Input: part model. Units: mm. Frame: model coordinates. A direction names the side the tool comes from. Round coordinates to 2 decimals unless told otherwise and drop trailing zeros. Loops run counter-clockwise (first coordinate to the right, second up) from the corner with the lowest first, then second, coordinate; pieces in that order, holes last. Notation, with made-up numbers: M 53.25,52 L 63.25,52 A8 ccw 63.25,60 Z; hole C -38.5,17 d6. An arc over 180 degrees is marked long. Use one line per item in the form item = value. Start each with the question number.
Q1. Ray query, line 1 along X through (y, z) = (0.75, -5.75); line 2 along Y through (x, z) = (4.25, 2); line 3 along Y through (x, z) = (-1, -2.5). Return the intervals inside material, ascending.
Q2. Section query D-D, the plane z = -0.85. Output: boundary loops of the cut face in (x, y), and give its area (3 significant figures).
Q3. Section query C-C, the plane y = 6.75. Output: boundary loops of the cut face in (x, z), and give its area (3 significant figures).
Q4. Mould query, pull axis X, two halves, no side actions, for faces 3 (the cylindrical face through (-7.134, 0.811, 5.536)), 4 (the flat face through (-2.5, 3, -1)), 5 (the flat face through (2, -0.01, 6)). Classes: pulls with the +X half, pulls with the -X half, needs draft (parallel to the pull), parting line crosses it, or undercut.
Q5. Access query for faces 1 (the flat face through (-7, -0.01, 6)), 2 (the flat face through (0, 3.6, -1)). Directions: +Z, -Z, +X, -X, +Y, -Y. A direction counts if a zero-diameter tool reaches every point of the face in a straight line with its end or side. Return the directions, or none.
Q6. Section query B-B, the plane z = -5.75. State how many separate pieces and enclosed holes the cut face has, and give its area (3 significant figures).
Q7. First-contact query: P1, Ø8.5, axis at x = 4.5, z = 2.5, coming from the +Y side; P2, Ø1.2, axis at x = 6.5, z = -6, coming from the +Y side; P3, Ø1.4, axis at x = -5, z = 6, coming from the +Y side; P4, Ø3, axis at x = 0, z = -5.5, coming from the -Y side. Flat tips, straight axial feed; report the tip coordinate or a pass-through.
```python
from build123d import *

# Parameters (mm, degrees)
BOSS_EXTRUDE1_DEPTH = 1.6
SKETCH2_R           = 1.1
SKETCH2_R_2         = 0.5
CUT_EXTRUDE1_DEPTH  = 1.6
SKETCH3_R           = 1.2
SKETCH3_R_2         = 1.09
SKETCH3_R_3         = 0.9
SKETCH3_R_4         = 0.49
BOSS_EXTRUDE2_DEPTH = 1.62
SKETCH5_W           = 5
SKETCH5_H           = 5
BOSS_EXTRUDE3_DEPTH = 2
SKETCH6_R           = 1.25
SKETCH6_R_2         = 0.95
BOSS_EXTRUDE4_DEPTH = 3.6


with BuildPart() as part:
    # Sketch1 → Boss-Extrude1 (new body)
    with BuildSketch(Plane(origin=(0, 0, 0), x_dir=(1, 0, 0), z_dir=(0, 1, 0))):
        with BuildLine():
            Line((-6.89, 8.35), (6.89, 8.35))
            ThreePointArc((6.89, 8.35), (8.304213562, 7.764213562), (8.89, 6.35))
            Line((8.89, 6.35), (8.89, -6.35))
            ThreePointArc((8.89, -6.35), (8.304213562, -7.764213562), (6.89, -8.35))
            Line((6.89, -8.35), (-6.89, -8.35))
            ThreePointArc((-6.89, -8.35), (-8.304213562, -7.764213562), (-8.89, -6.35))
            Line((-8.89, -6.35), (-8.89, 6.35))
            ThreePointArc((-8.89, 6.35), (-8.304213562, 7.764213562), (-6.89, 8.35))
        make_face()
    extrude(amount=BOSS_EXTRUDE1_DEPTH)

    # Sketch2 → Cut-Extrude1 (cut)
    with BuildSketch(Plane(origin=(0, 1.6, 0), x_dir=(1, 0, 0), z_dir=(0, 1, 0))):
        with Locations(Location((-6.29, 5.75, 0), (0, 0, 270))):
            Circle(SKETCH2_R)
        with Locations(Location((6.29, 5.75, 0), (0, 0, 90))):
            Circle(SKETCH2_R)
        with Locations(Location((-7.62, -5.6, 0), (0, 0, 270))):
            Circle(SKETCH2_R_2)
        with Locations(Location((-5.08, -5.6, 0), (0, 0, 270))):
            Circle(SKETCH2_R_2)
        with Locations(Location((-2.54, -5.6, 0), (0, 0, 270))):
            Circle(SKETCH2_R_2)
        with Locations(Location((0, -5.6, 0), (0, 0, 270))):
            Circle(SKETCH2_R_2)
        with Locations(Location((2.54, -5.6, 0), (0, 0, 270))):
            Circle(SKETCH2_R_2)
        with Locations(Location((5.08, -5.6, 0), (0, 0, 270))):
            Circle(SKETCH2_R_2)
        with Locations(Location((7.62, -5.6, 0), (0, 0, 270))):
            Circle(SKETCH2_R_2)
    extrude(amount=-CUT_EXTRUDE1_DEPTH, mode=Mode.SUBTRACT)

    # Sketch3 → Boss-Extrude2 (add)
    # profile 1 of 9: a face of its own
    with BuildSketch(Plane(origin=(0, 1.61, 0), x_dir=(1, 0, 0), z_dir=(0, 1, 0))):
        with Locations(Location((-6.29, 5.75, 0), (0, 0, 270))):
            Circle(SKETCH3_R)
        with Locations(Location((-6.29, 5.75, 0), (0, 0, 270))):
            Circle(SKETCH3_R_2, mode=Mode.SUBTRACT)
    # profile 2 of 9: a face of its own
    with BuildSketch(Plane(origin=(0, 1.61, 0), x_dir=(1, 0, 0), z_dir=(0, 1, 0))):
        with Locations(Location((6.29, 5.75, 0), (0, 0, 270))):
            Circle(SKETCH3_R)
        with Locations(Location((6.29, 5.75, 0), (0, 0, 270))):
            Circle(SKETCH3_R_2, mode=Mode.SUBTRACT)
    # profile 3 of 9: a face of its own
    with BuildSketch(Plane(origin=(0, 1.61, 0), x_dir=(1, 0, 0), z_dir=(0, 1, 0))):
        with Locations(Location((7.62, -5.6, 0), (0, 0, 270))):
            Circle(SKETCH3_R_3)
        with Locations(Location((7.62, -5.6, 0), (0, 0, 270))):
            Circle(SKETCH3_R_4, mode=Mode.SUBTRACT)
    # profile 4 of 9: a face of its own
    with BuildSketch(Plane(origin=(0, 1.61, 0), x_dir=(1, 0, 0), z_dir=(0, 1, 0))):
        with Locations(Location((5.08, -5.6, 0), (0, 0, 270))):
            Circle(SKETCH3_R_3)
        with Locations(Location((5.08, -5.6, 0), (0, 0, 270))):
            Circle(SKETCH3_R_4, mode=Mode.SUBTRACT)
    # profile 5 of 9: a face of its own
    with BuildSketch(Plane(origin=(0, 1.61, 0), x_dir=(1, 0, 0), z_dir=(0, 1, 0))):
        with Locations(Location((2.54, -5.6, 0), (0, 0, 270))):
            Circle(SKETCH3_R_3)
        with Locations(Location((2.54, -5.6, 0), (0, 0, 270))):
            Circle(SKETCH3_R_4, mode=Mode.SUBTRACT)
    # profile 6 of 9: a face of its own
    with BuildSketch(Plane(origin=(0, 1.61, 0), x_dir=(1, 0, 0), z_dir=(0, 1, 0))):
        with Locations(Location((0, -5.6, 0), (0, 0, 270))):
            Circle(SKETCH3_R_3)
        with Locations(Location((0, -5.6, 0), (0, 0, 270))):
            Circle(SKETCH3_R_4, mode=Mode.SUBTRACT)
    # profile 7 of 9: a face of its own
    with BuildSketch(Plane(origin=(0, 1.61, 0), x_dir=(1, 0, 0), z_dir=(0, 1, 0))):
        with Locations(Location((-2.54, -5.6, 0), (0, 0, 270))):
            Circle(SKETCH3_R_3)
        with Locations(Location((-2.54, -5.6, 0), (0, 0, 270))):
            Circle(SKETCH3_R_4, mode=Mode.SUBTRACT)
    # profile 8 of 9: a face of its own
    with BuildSketch(Plane(origin=(0, 1.61, 0), x_dir=(1, 0, 0), z_dir=(0, 1, 0))):
        with Locations(Location((-5.08, -5.6, 0), (0, 0, 270))):
            Circle(SKETCH3_R_3)
        with Locations(Location((-5.08, -5.6, 0), (0, 0, 270))):
            Circle(SKETCH3_R_4, mode=Mode.SUBTRACT)
    # profile 9 of 9: a face of its own
    with BuildSketch(Plane(origin=(0, 1.61, 0), x_dir=(1, 0, 0), z_dir=(0, 1, 0))):
        with Locations(Location((-7.62, -5.6, 0), (0, 0, 270))):
            Circle(SKETCH3_R_3)
        with Locations(Location((-7.62, -5.6, 0), (0, 0, 270))):
            Circle(SKETCH3_R_4, mode=Mode.SUBTRACT)
    extrude(amount=-BOSS_EXTRUDE2_DEPTH)

    # Sketch5 → Boss-Extrude3 (add)
    with BuildSketch(Plane(origin=(0, 1.6, 0), x_dir=(1, 0, 0), z_dir=(0, 1, 0))):
        with Locations((0, 0.85)):
            Rectangle(SKETCH5_W, SKETCH5_H)
    extrude(amount=BOSS_EXTRUDE3_DEPTH)

    # Sketch6 → Boss-Extrude4 (add)
    with BuildSketch(Plane(origin=(0, 3.6, 0), x_dir=(1, 0, 0), z_dir=(0, 1, 0))):
        with Locations(Location((0, 0.85, 0), (0, 0, 270))):
            Circle(SKETCH6_R)
        with Locations(Location((0, 0.85, 0), (0, 0, 270))):
            Circle(SKETCH6_R_2, mode=Mode.SUBTRACT)
    extrude(amount=BOSS_EXTRUDE4_DEPTH)


solid = part.part
```
Results found:
q1.line_1 = -8.89 to -7.38, -5.2 to 5.2, 7.38 to 8.89
q1.line_2 = 0 to 1.6
q1.line_3 = 0 to 3.6
q2.outline = M -8.89,0 L 8.89,0 L 8.89,1.6 L 2.5,1.6 L 2.5,3.6 L 1.25,3.6 L 1.25,7.2 L 0.95,7.2 L 0.95,3.6 L -0.95,3.6 L -0.95,7.2 L -1.25,7.2 L -1.25,3.6 L -2.5,3.6 L -2.5,1.6 L -8.89,1.6 Z
q2.area = 40.6 mm²
q3.outline = C 0,-0.85 d2.5; hole C 0,-0.85 d1.9
q3.area = 2.07 mm²
q4.face_3 = undercut
q4.face_4 = pulls with the -X half
q4.face_5 = needs draft
q5.face_1 = +Z, -Z, +X, -X, -Y
q5.face_2 = +Y
q6.separate_pieces = 3
q6.enclosed_holes = 0
q6.area = 21.5 mm²
q7.P1 = 3.6
q7.P2 = through
q7.P3 = 1.61
q7.P4 = 0
